Can you work these out from the model? Positions are in its coordinate system, mm. Face numbers are marked on the shaded views. A direction names the side the tool comes from. Give positions to 0.01 mm unless a question says otherwise; leave off trailing zeros. Write each loop counter-clockwise with the first axis right and the second up, starting at its lowest first coordinate (ties: lowest second). Pieces come first, ordered by that corner, then holes. Notation, with made-up numbers: (75, -5) - (131, -5) arc R11 ccw to (131, 1) - close; hole circle Ø4 at (11.25, 12). An arc over 180 degrees is marked (long way). Use a Markdown table: item, result. Add a question column.
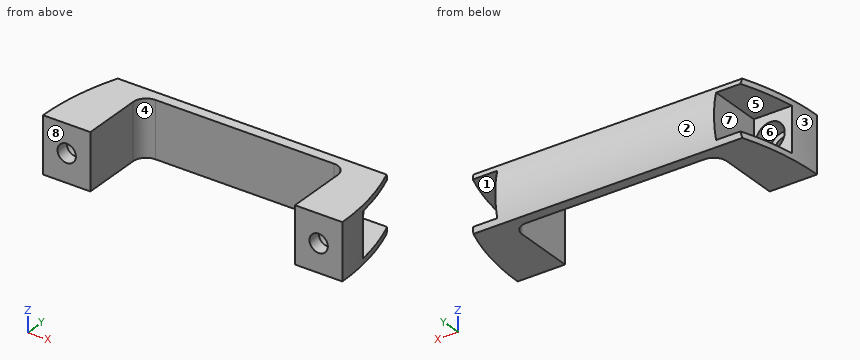
Autodesk Inventor part; units mm, degrees
ref_plane "handle_to_body_XY" through (58.5, 0, 0) normal (0, 1, 0) x (1, 0, 0)
ref_plane "handle_to_body_YZ" through (58.5, 0, 0) normal (1, 0, 0) x (0, 0, -1)
ref_plane "handle_to_body_ZX" through (58.5, 0, 0) normal (0, 0, -1) x (0, 1, 0)
sketch "Sketch_1" plane through (0, 0, 0) normal (0, 0, 1) x (1, 0, 0)
  line L0 (-11, 0) -> (11, 0)
  line L1 (11, 0) -> (11, 28)
  arc A0 (17, 34) -> (11, 28) centre (17, 28) ccw
  line L2 (17, 34) -> (100, 34)
  arc A1 (106, 28) -> (100, 34) centre (100, 28) ccw
  line L3 (106, 28) -> (106, 0)
  line L4 (106, 0) -> (128, 0)
  arc A2 (128, 0) -> (120.8624, 39.061) centre (17.55, 0) ccw
  arc A3 (120.8624, 39.061) -> (118.0562, 41) centre (118.0562, 38) ccw
  line L5 (118.0562, 41) -> (-1.0562, 41)
  arc A4 (-1.0562, 41) -> (-3.8624, 39.061) centre (-1.0562, 38) ccw
  arc A5 (-3.8624, 39.061) -> (-11, 0) centre (99.45, 0) ccw
extrude "Extrusion1" add sketch "Sketch_1" along normal mid plane 26
sketch "Sketch_2" plane through (0, 15, 0) normal (0, 1, 0) x (1, 0, 0)
  line L0 (-58.5, -26) -> (175.5, -26)
  line L1 (175.5, -26) -> (175.5, 26)
  line L2 (175.5, 26) -> (-58.5, 26)
  line L3 (-58.5, 26) -> (-58.5, -26)
  line L4 (-11, 10.4) -> (7.7, 10.4)
  line L5 (7.7, 10.4) -> (7.7, -10.4)
  line L6 (7.7, -10.4) -> (-11, -10.4)
  line L7 (-11, -10.4) -> (-11, -13)
  line L8 (-11, -13) -> (128, -13)
  line L9 (128, -13) -> (128, -10.4)
  line L10 (128, -10.4) -> (109.3, -10.4)
  line L11 (109.3, -10.4) -> (109.3, 10.4)
  line L12 (109.3, 10.4) -> (128, 10.4)
  line L13 (128, 10.4) -> (128, 13)
  line L14 (128, 13) -> (-11, 13)
  line L15 (-11, 13) -> (-11, 10.4)
extrude "Extrusion2" cut sketch "Sketch_2" along normal blind 58.5
sketch "Sketch3" plane through (0, 15, 0) normal (0, 1, 0) x (1, 0, 0)
  point P0 (0, 0)
hole "Hole1" at (0, 15, 0) direction (0, -1, 0) diameter 8.5 depth 15 counterbore diameter 13.3 counterbore depth 9
sketch "Sketch4" plane through (0, 15, 0) normal (0, 1, 0) x (1, 0, 0)
  point P0 (117, 0)
hole "Hole2" at (117, 15, 0) direction (0, -1, 0) diameter 8.5 depth 15 counterbore diameter 13.3 counterbore depth 9
sketch "Sketch_6" plane through (-11, 0, 0) normal (1, 0, 0) x (0, 0, -1)
  line L0 (-13, 46) -> (-13, 38.8844)
  arc A0 (13, 38.8844) -> (-13, 38.8844) centre (0, 0) ccw
  line L1 (13, 38.8844) -> (13, 46)
  line L2 (13, 46) -> (-13, 46)
extrude "Extrusion3" cut sketch "Sketch_6" along normal blind 139
ref_plane "handle_to_body_XY" through (58.5, 0, 0) normal (0, 1, 0) x (1, 0, 0)
ref_plane "handle_to_body_YZ" through (58.5, 0, 0) normal (1, 0, 0) x (0, 0, -1)
ref_plane "handle_to_body_ZX" through (58.5, 0, 0) normal (0, 0, -1) x (0, 1, 0)
ref_plane "handle_to_bolt1_XY" through (117, 6, 0) normal (0, 1, 0) x (1, 0, 0)
ref_plane "handle_to_bolt1_YZ" through (117, 6, 0) normal (1, 0, 0) x (0, 0, -1)
ref_plane "handle_to_bolt1_ZX" through (117, 6, 0) normal (0, 0, -1) x (0, 1, 0)
ref_plane "handle_to_bolt2_XY" through (0, 6, 0) normal (0, 1, 0) x (1, 0, 0)
ref_plane "handle_to_bolt2_YZ" through (0, 6, 0) normal (1, 0, 0) x (0, 0, -1)
ref_plane "handle_to_bolt2_ZX" through (0, 6, 0) normal (0, 0, -1) x (0, 1, 0)
ref_plane "handle_to_nut1_XY" through (117, 0, 0) normal (0, 1, 0) x (1, 0, 0)
ref_plane "handle_to_nut1_YZ" through (117, 0, 0) normal (1, 0, 0) x (0, 0, -1)
ref_plane "handle_to_nut1_ZX" through (117, 0, 0) normal (0, 0, -1) x (0, 1, 0)
ref_plane "handle_to_nut2_XY" through (0, 0, 0) normal (0, 1, 0) x (1, 0, 0)
ref_plane "handle_to_nut2_YZ" through (0, 0, 0) normal (1, 0, 0) x (0, 0, -1)
ref_plane "handle_to_nut2_ZX" through (0, 0, 0) normal (0, 0, -1) x (0, 1, 0)
ref_plane "to_nut_1_XY" through (0, -5.5, 0) normal (0, -1, 0) x (1, 0, 0)
ref_plane "to_nut_1_YZ" through (0, -5.5, 0) normal (1, 0, 0) x (0, 0, 1)
ref_plane "to_nut_1_ZX" through (0, -5.5, 0) normal (0, 0, 1) x (0, -1, 0)
ref_plane "to_nut_2_XY" through (117, -5.5, 0) normal (0, -1, 0) x (1, 0, 0)
ref_plane "to_nut_2_YZ" through (117, -5.5, 0) normal (1, 0, 0) x (0, 0, 1)
ref_plane "to_nut_2_ZX" through (117, -5.5, 0) normal (0, 0, 1) x (0, -1, 0)
properties part number "UPCN26-B-41"
Q1. Suppose I cut it at D-D (y = 12). Please give me the cut outline in (x, z), and give its area (3 significant figures).
Q2. If we mould it in two halves opening along X, with no side actions, what happens to the marked faces 6, 7 and 8? For each: released by +X, released by -X, zero draft, split by the parting line, or undercut.
Q3. I'm going to push flat-ended pins straight in: P1, Ø3, axis at x = 38.5, z = -4.5, coming from the -Y side; P2, Ø13.5, axis at x = 0, z = 0, coming from the +Y side; P3, Ø3, axis at y = 37, z = 4, coming from the +X side. Where does each tip first touch, or does it pass through?
Q4. If I drill on probe 1 along Z at (x, y) = (117, 7); probe 2 along Z at (x, y) = (0, 2.1); probe 3 along X at (y, z) = (19.5, 1.75), over which ranges is the centre line in solid material (lowest first)? Write a range as [from, to].
Q5. On a 3-axis mill with a long thin cutter (end or side, diameter ignored), from which of +Z, -Z, +X, -X, +Y, -Y can I reach the whole of each face in a straight line? I mean the marked faces 1, 2, 3, 4 and 5. Say none if no direction works.
Q6. Suppose I cut it at B-B (x = 117). Please give me the cut outline in (y, z).
Q7. Suppose I cut it at C-C (y = 23). Please give me the cut outline in (x, z).
Q8. Suppose I cut it at A-A (z = 0). Give the number of separate pieces and of enclosed holes in the cut face, and give its area (3 significant figures).
Derived:
| question | item | result |
|---|---|---|
| 1 | outline | (-10.35, -13) - (11, -13) - (11, 13) - (-10.35, 13) - close; (106, -13) - (127.35, -13) - (127.35, 13) - (106, 13) - close; hole circle Ø13.3 at (0, 0); hole circle Ø13.3 at (117, 0) |
| 1 | area | 832 mm² |
| 2 | face 6 | undercut |
| 2 | face 7 | released by -X |
| 2 | face 8 | zero draft |
| 3 | P1 | y = 34 |
| 3 | P2 | y = 15 |
| 3 | P3 | x = 109.3 |
| 4 | probe 1 | [-13, -6.65], [6.65, 13] |
| 4 | probe 2 | [-13, -4.25], [4.25, 13] |
| 4 | probe 3 | [7.7, 11], [106, 109.3] |
| 5 | face 1 | +X, +Y |
| 5 | face 2 | +X, -X, +Y |
| 5 | face 3 | +Z, -Z, -X, +Y |
| 5 | face 4 | +Z, -Z, -Y |
| 5 | face 5 | -X, +Y |
| 6 | outline | (0, -13) - (38.88, -13) arc R41 ccw to (39.66, -10.4) - (15, -10.4) - (15, -6.65) - (6, -6.65) - (6, -4.25) - (0, -4.25) - close; (0, 4.25) - (6, 4.25) - (6, 6.65) - (15, 6.65) - (15, 10.4) - (39.66, 10.4) arc R41 ccw to (38.88, 13) - (0, 13) - close |
| 7 | outline | (-8.58, -13) - (11, -13) - (11, 13) - (-8.58, 13) - (-8.58, 10.4) - (7.7, 10.4) - (7.7, -10.4) - (-8.58, -10.4) - close; (106, -13) - (125.58, -13) - (125.58, -10.4) - (109.3, -10.4) - (109.3, 10.4) - (125.58, 10.4) - (125.58, 13) - (106, 13) - close |
| 8 | separate pieces | 3 |
| 8 | enclosed holes | 0 |
| 8 | area | 1,160 mm² |
